```python
from build123d import *

# Parameters (mm, degrees)
ESBO_O1_R                 = 0.5
RESSALTO_EXTRUS_O1_DEPTH  = 1.6
FILETE1_R                 = 10
ESBO_O2_R                 = 1.5
CORTE_EXTRUS_O1_DEPTH     = 119.14439181
ESPELHAR2_COPY_1_SKETCH_R = 1.5
ESPELHAR2_COPY_1_DEPTH    = 119.14439181


with BuildPart() as part:
    # Esboço1 → Ressalto-extrusão1 (new body)
    with BuildSketch(Plane(origin=(0, 0, 0), x_dir=(1, 0, 0), z_dir=(0, 1, 0))):
        with BuildLine():
            ThreePointArc((68.191990862, -68.984435798), (89.508723356, -37.378983978), (97, 0))
            ThreePointArc((97, 0), (89.508723356, 37.378983978), (68.191990862, 68.984435798))
            ThreePointArc((68.191990862, 68.984435798), (0, 57), (-68.191990862, 68.984435798))
            ThreePointArc((-68.191990862, 68.984435798), (-97, 0), (-68.191990862, -68.984435798))
            ThreePointArc((-68.191990862, -68.984435798), (0, -57), (68.191990862, -68.984435798))
        make_face()
        with Locations(Location((0, 0, 0), (0, 0, 270))):
            Circle(ESBO_O1_R, mode=Mode.SUBTRACT)
    extrude(amount=RESSALTO_EXTRUS_O1_DEPTH)

    # Filete1
    filete1_edges = [part.edges().sort_by_distance(p)[0] for p in [
        (-68.191990862, 0.8, -68.984435798),
        (68.191990862, 0.8, -68.984435798),
        (68.191990862, 0.8, 68.984435798),
        (-68.191990862, 0.8, 68.984435798),
    ]]
    fillet(filete1_edges, radius=FILETE1_R)

    # Esboço2 → Corte-extrusão1 (cut, through all)
    with BuildSketch(Plane(origin=(0, 1.6, 0), x_dir=(1, 0, 0), z_dir=(0, 1, 0))):
        with Locations(Location((-50, 55, 0), (0, 0, 270))):
            Circle(ESBO_O2_R)
    corte_extrus_o1 = extrude(amount=-CORTE_EXTRUS_O1_DEPTH, mode=Mode.SUBTRACT)

    # Espelhar1: Corte-extrusão1 across plane
    add(corte_extrus_o1.mirror(Plane(origin=(0, 0, 0), x_dir=(0, 0, 1), z_dir=(1, 0, 0))), mode=Mode.SUBTRACT)

    # Espelhar2: Corte-extrusão1 across plane
    add(corte_extrus_o1.mirror(Plane.XY), mode=Mode.SUBTRACT)

    # Espelhar2 copy 1 sketch → Espelhar2 copy 1 (cut, through all)
    with BuildSketch(Plane(origin=(0, 1.6, 0), x_dir=(-1, 0, 0), z_dir=(0, 1, 0))):
        with Locations(Location((-50, 55, 0), (0, 0, 270))):
            Circle(ESPELHAR2_COPY_1_SKETCH_R)
    extrude(amount=-ESPELHAR2_COPY_1_DEPTH, mode=Mode.SUBTRACT)


solid = part.part
```
Could you check a few things on this model? Use its own coordinates, in mm. Coordinates: 2 decimals unless noted, no trailing zeros. Order: outer loops, then holes, each group sorted by start corner. A loop starts at its lowest first (then second) coordinate and runs counter-clockwise, first axis right, second up. Notation, with made-up numbers: M 13,-40 L 67,-40 A31 ccw 67,-16 Z; hole C 38.5,-7.5 d3. An arc over 180 degrees is marked long. Use a Markdown table: item, result. Add a question column.
Q1. I want a section at C-C on x = -59. List the corners of the cut face in (y, z) for me, then the cut area to 3 significant figures.
Q2. I'm going to push a flat-ended pin straight in: pin 1 (1.8 mm diameter, centred on x = 50, z = 55, fed in from +Y). Where does the tip first touch, or does it pass through?
Q3. If I drill on L1, parallel to Z at x = 50, y = 0.65; L2, parallel to X at y = 0.85, z = 55; L3, parallel to Z at x = -50.5, y = 1, over which ranges is the centre line in solid material (lowest first)?
Q4. I want a section at A-A on y = 0.5. Give the number of separate pieces and of enclosed holes in the cut face, then the cut area to 3 significant figures.
Q5. We'd pull the mould along X, two halves only. Please class faces 1 (the cylindrical face through (-96.995, 0.789, -0.979)), 2 (the flat face through (-1, 0, -1)), 3 (the cylindrical face through (-0.89, 0.79, 57)): pulls with the +X half, pulls with the -X half, needs draft (parallel to the pull), parting line crosses it, or undercut.
Q6. I want a section at B-B on z = -43. List the corners of the cut face in (x, y) for me, then the cut area to 3 significant figures.
Checked values:
| question | item | result |
|---|---|---|
| 1 | outline | M 0,-65.9 L 1.6,-65.9 L 1.6,65.9 L 0,65.9 Z |
| 1 | area | 211 mm² |
| 2 | pin 1 | through |
| 3 | L1 | -63.35 to -56.5, -53.5 to 53.5, 56.5 to 63.35 |
| 3 | L2 | -79.9 to -51.5, -48.5 to 48.5, 51.5 to 79.9 |
| 3 | L3 | -63.48 to -56.41, -53.59 to 53.59, 56.41 to 63.48 |
| 4 | separate pieces | 1 |
| 4 | enclosed holes | 5 |
| 4 | area | 22,000 mm² |
| 5 | face 1 | pulls with the -X half |
| 5 | face 2 | needs draft |
| 5 | face 3 | undercut |
| 6 | outline | M -86.95,0 L 86.95,0 L 86.95,1.6 L -86.95,1.6 Z |
| 6 | area | 278 mm² |
